Build history of the part. All positions in model axes, mm. A direction names the side the tool comes from. Give positions to 0.01 mm unless a question says otherwise; leave off trailing zeros. Order: outer loops, then holes, each group sorted by start corner. A loop starts at its lowest first (then second) coordinate and runs counter-clockwise, first axis right, second up. Notation, with made-up numbers: (-16.5, -16.75) -> (29.5, -16.75) arc R22 cw to (29.5, 14.25) -> close; hole circle Ø3 at (7, 60). An arc over 180 degrees is marked (long way). Write item = value, one per line. Start each with the question number.
from build123d import *

# Parameters (mm, degrees)
F0_W     = 25.4
F0_H     = 25.4
F1_DEPTH = 25.4


with BuildPart() as f1:
    # F0 (on Front) → F1 (new body)
    with BuildSketch(Plane.XZ):
        with Locations((-25.4, 25.4)):
            Rectangle(F0_W, F0_H)
        with Locations((0, 25.4)):
            Rectangle(F0_W, F0_H)
        with Locations((25.4, 25.4)):
            Rectangle(F0_W, F0_H)
        with Locations((25.4, 0)):
            Rectangle(F0_W, F0_H)
        with Locations((25.4, -25.4)):
            Rectangle(F0_W, F0_H)
        with Locations((0, -25.4)):
            Rectangle(F0_W, F0_H)
        with Locations((-25.4, -25.4)):
            Rectangle(F0_W, F0_H)
        with Locations((-25.4, 0)):
            Rectangle(F0_W, F0_H)
    extrude(amount=F1_DEPTH)


solid = f1.part
(1) Cut at C-C, the plane y = -9.25. Give the cut face in (x, z), plus the area to 3 significant figures.
(2) 3-axis set-ups, long thin cutter, end or side, ignore diameter. For faces 1 (the face through (16, -25.4, 1)), 2 (the face through (-12.7, -13, 0)): which of +Z, -Z, +X, -X, +Y, -Y reach the whole face in a straight line?
(3) Cut at A-A, the plane x = -10. Give the cut face in (y, z), plus the area to 3 significant figures.
(4) Wall check: line 1 (X direction, y = -20.5, z = 7). Give the ranges that are in metal, low to high. Write a range as [from, to].
(5) Cut at B-B, the plane z = -6. Give the cut face in (x, y).
(6) Mould opens along Z. For faces 3 (the face through (1, -13, 38.1)), 4 (the face through (0, -13, -12.7)), 5 (the face through (16, 0, 1)), 6 (the face through (-1, -13, -38.1)) say: released by +Z, released by -Z, zero draft, split by the parting line, or undercut.
Results:
q1.outline = (-38.1, -38.1) -> (38.1, -38.1) -> (38.1, 38.1) -> (-38.1, 38.1) -> close; hole (-12.7, -12.7) -> (12.7, -12.7) -> (12.7, 12.7) -> (-12.7, 12.7) -> close
q1.area = 5,160 mm2
q2.face_1 = +Z, -Z, +X, -X, -Y
q2.face_2 = +Y, -Y
q3.outline = (-25.4, -38.1) -> (0, -38.1) -> (0, -12.7) -> (-25.4, -12.7) -> close; (-25.4, 12.7) -> (0, 12.7) -> (0, 38.1) -> (-25.4, 38.1) -> close
q3.area = 1,290 mm2
q4.line_1 = [-38.1, -12.7], [12.7, 38.1]
q5.outline = (-38.1, -25.4) -> (-12.7, -25.4) -> (-12.7, 0) -> (-38.1, 0) -> close; (12.7, -25.4) -> (38.1, -25.4) -> (38.1, 0) -> (12.7, 0) -> close
q6.face_3 = released by +Z
q6.face_4 = undercut
q6.face_5 = zero draft
q6.face_6 = released by -Z
